The drawing under review shows one solid part. Ordinate dimensions are in mm from its lowest x, y, z. A direction names the side the tool comes from. Coordinates: 2 decimals unless noted, no trailing zeros. Loops run counter-clockwise (first coordinate to the right, second up) from the corner with the lowest first, then second, coordinate; pieces in that order, holes last. Notation, with made-up numbers: M -19,30 L 6,30 A30 cw 6,67 Z; hole C 80.25,88 d8. An arc over 180 degrees is marked long. Answer as CSV lines item,"result". Start each with the question number.
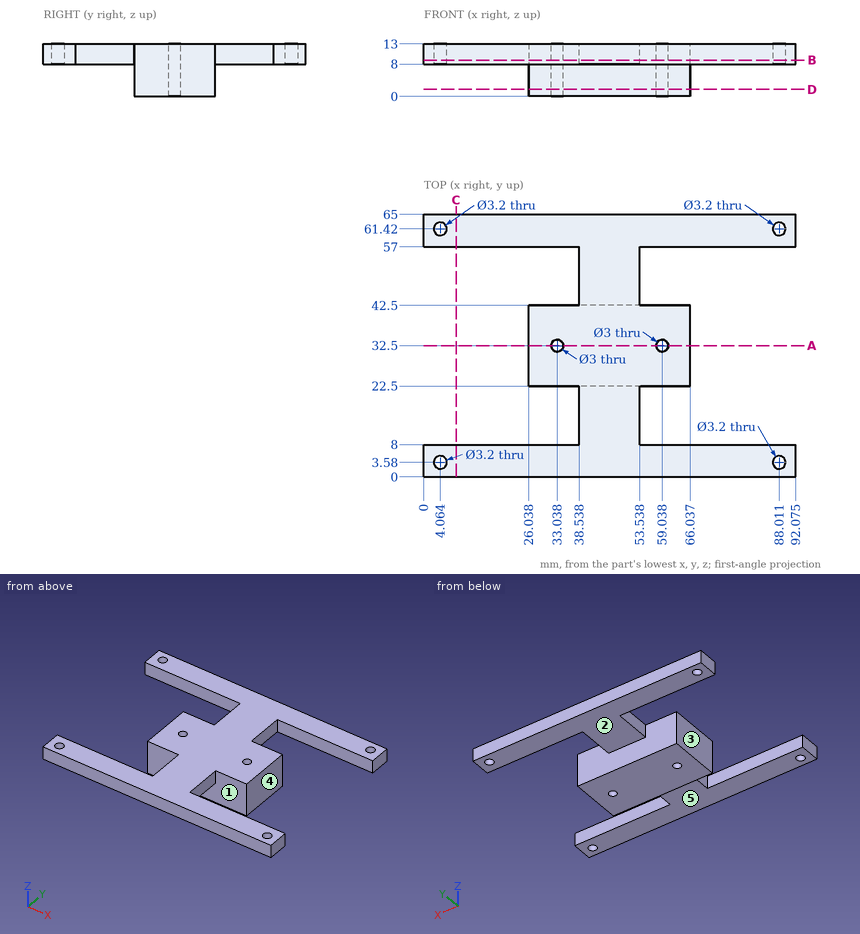
Item 1: Mouldability with a two-part tool opening along Y and no side actions: class the marked faces 4 and 5 as released by +Y, released by -Y, zero draft, split by the parting line, or undercut.
Item 2: For line 1 along Y through (x, z) = (36.5, 12.75); line 2 along X through (y, z) = (32.5, 8); line 3 along Y through (x, z) = (86, 12), list the stretches that pass through material, from the lowest coordinate up. Write a range as from..to.
Item 3: For pin 1 (1.5 mm diameter, centred on y = 52.5, z = 11, fed in from +X); pin 2 (1.8 mm diameter, centred on x = 33.04, y = 32.5, fed in from +Z); pin 3 (4 mm diameter, centred on x = 36, z = 5, fed in from -Y); pin 4 (6 mm diameter, centred on y = 37, z = 2.5, fed in from -X), all flat-tipped, find the tip position at first contact; note any pin that passes through.
Item 4: For the marked faces 1, 2 and 3, list the 3-axis set-ups (+Z, -Z, +X, -X, +Y, -Y) from which the entire face can be reached by the end or side of a thin tool; tool diameter is ignored.
Item 5: Add section C-C (x = 8). Give the boundary of the cut face in (y, z).
Item 6: Add section B-B (z = 9). Give the boundary of the cut face in (x, y) (1 decimal).
Item 7: Add section A-A (y = 32.5). Give the boundary of the cut face in (x, z).
Item 8: Add section D-D (z = 1.75). Give the boundary of the cut face in (x, y).
Response:
1,face 4,"undercut"
1,face 5,"zero draft"
2,line 1,"0..8, 22.5..42.5, 57..65"
2,line 2,"26.04..31.54, 34.54..57.54, 60.54..66.04"
2,line 3,"0..8, 57..65"
3,pin 1,"x = 53.54"
3,pin 2,"through"
3,pin 3,"y = 22.5"
3,pin 4,"x = 26.04"
4,face 1,"-Z"
4,face 2,"-Z, +X, -X, +Y"
4,face 3,"+Z, -Z, -X"
5,outline,"M 0,8 L 8,8 L 8,13 L 0,13 Z; M 57,8 L 65,8 L 65,13 L 57,13 Z"
6,outline,"M 0,0 L 92.1,0 L 92.1,8 L 53.5,8 L 53.5,22.5 L 66,22.5 L 66,42.5 L 53.5,42.5 L 53.5,57 L 92.1,57 L 92.1,65 L 0,65 L 0,57 L 38.5,57 L 38.5,42.5 L 26,42.5 L 26,22.5 L 38.5,22.5 L 38.5,8 L 0,8 Z; hole C 4.1,3.6 d3.2; hole C 4.1,61.4 d3.2; hole C 33,32.5 d3; hole C 59,32.5 d3; hole C 88,3.6 d3.2; hole C 88,61.4 d3.2"
7,outline,"M 26.04,0 L 31.54,0 L 31.54,13 L 26.04,13 Z; M 34.54,0 L 57.54,0 L 57.54,13 L 34.54,13 Z; M 60.54,0 L 66.04,0 L 66.04,13 L 60.54,13 Z"
8,outline,"M 26.04,22.5 L 66.04,22.5 L 66.04,42.5 L 26.04,42.5 Z; hole C 33.04,32.5 d3; hole C 59.04,32.5 d3"
